Can you work these out from the model? Positions are in its coordinate system, mm. Coordinates: 2 decimals unless noted, no trailing zeros. Loops run counter-clockwise (first coordinate to the right, second up) from the corner with the lowest first, then second, coordinate; pieces in that order, holes last. Notation, with made-up numbers: (26.5, 63.25) -> (85.5, 63.25) arc R13 cw to (85.5, 80.25) -> close; hole circle Ø6 at (76, 36.5). An arc over 180 degrees is marked (long way). Use one line per item in the form item = value. Start each with the question number.
(1) I'm going to push flat-ended pins straight in: pin 1 (1 mm diameter, centred on x = -11, z = -14.5, fed in from +Y); pin 2 (2 mm diameter, centred on y = -266, z = -11.5, fed in from +X); pin 3 (1 mm diameter, centred on x = -0.5, z = -6, fed in from -Y); pin 4 (4 mm diameter, centred on x = -16, y = -855.5, fed in from -Z). Where does each tip first touch, or does it pass through?
(2) Imagine slicing it at A-A (y = -794). List the corners of the cut face in (x, z) for me, plus the area to 3 significant figures.
(3) I need wall thicknesses on line 1 (Z direction, x = 0, y = -1023); line 2 (X direction, y = -277, z = -1.5); line 3 (X direction, y = -394.5, z = 1). Which ranges of each line are inside material? Lowest first, please. Write a range as [from, to].
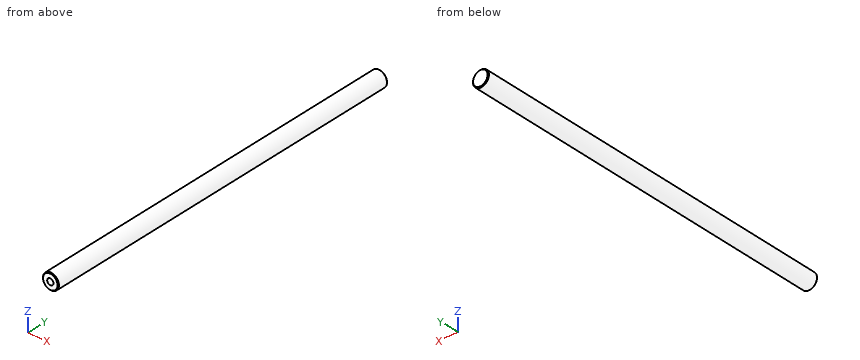
```python
from build123d import *

# Parameters (mm, degrees)
F0_R     = 22.5
F1_DEPTH = 1040
F2_SIZE  = 2
F4_D     = 17.5
F4_DEPTH = 35
F4_TIP   = 5.2575304165


with BuildPart() as f1:
    # F0 (on Front) → F1 (new body)
    with BuildSketch(Plane.XZ):
        Circle(F0_R)
    extrude(amount=F1_DEPTH)

    # F2
    f2_edges = [f1.edges().sort_by_distance(p)[0] for p in [
        (-22.5, 0, 0),
        (-22.5, -1040, 0),
    ]]
    chamfer(f2_edges, length=F2_SIZE)

    # F4
    with Locations(Plane.XZ.offset(1040)):
        with Locations((0, 0)):
            Hole(F4_D / 2, depth=F4_DEPTH)
            with Locations((0, 0, -(F4_DEPTH + F4_TIP / 2))):  # 118° drill point
                Cone(0, F4_D / 2, F4_TIP, mode=Mode.SUBTRACT)


solid = f1.part
```
Worked out:
q1.pin_1 = 0
q1.pin_2 = 19.9
q1.pin_3 = -1003.66
q1.pin_4 = -17.61
q2.outline = circle Ø45 at (0, 0)
q2.area = 1,590 mm2
q3.line_1 = [-22.5, -8.75], [8.75, 22.5]
q3.line_2 = [-22.45, 22.45]
q3.line_3 = [-22.48, 22.48]
